from build123d import *

# Parameters (mm, degrees)
F0_W     = 1.5
F0_H     = 2
F0_H_2   = 1.5
F0_W_2   = 6.5
F0_W_3   = 9.5
F1_DEPTH = 89
F2_R     = 1.25
F3_DEPTH = 25


with BuildPart() as f1:
    # F0 (on Front) → F1 (new body)
    with BuildSketch(Plane.XZ):
        with Locations((3.25, -1.75)):
            Rectangle(F0_W, F0_H)
        with Locations((3.25, 0)):
            Rectangle(F0_W, F0_H_2)
        Polygon((4.75, -1.75), (4, -0.75), (4, -2.75), align=None)
        with Locations((-0.75, 0)):
            Rectangle(F0_W_2, F0_H_2)
        with Locations((8.75, -3.5)):
            Rectangle(F0_W_3, F0_H_2)
        with Locations((3.25, -3.5)):
            Rectangle(F0_W, F0_H_2)
        with Locations((14.25, -1.75)):
            Rectangle(F0_W, F0_H)
        with Locations((14.25, -3.5)):
            Rectangle(F0_W, F0_H_2)
        Polygon((12.75, -1.75), (13.5, -2.75), (13.5, -0.75), align=None)
    extrude(amount=-F1_DEPTH)

    # F2 (on face) → F3 (cut)
    with BuildSketch(Plane.XY.offset(0.75)):
        with Locations((0, 4)):
            Circle(F2_R)
        with Locations((0, 85)):
            Circle(F2_R)
    extrude(amount=-F3_DEPTH, mode=Mode.SUBTRACT)


solid = f1.part
Can you work these out from the model? Positions are in its coordinate system, mm. A direction names the side the tool comes from. Round coordinates to 2 decimals unless told otherwise and drop trailing zeros. Write each loop counter-clockwise with the first axis right and the second up, starting at its lowest first coordinate (ties: lowest second). Pieces come first, ordered by that corner, then holes. Notation, with made-up numbers: (62, 7.5) -> (110, 7.5) arc R16 ccw to (110, 18.5) -> close; hole circle Ø7 at (9, -14). An arc over 180 degrees is marked (long way). Use one line per item in the form item = value. Start each with the question number.
Q1. Which directions (+Z, -Z, +X, -X, +Y, -Y) give clear straight access to the entire face, cutting with the end or side of a thin tool? Please do faces 4 (the face through (2.5, 44, -2)), 5 (the face through (5, 0, -3)), 6 (the face through (4, 44, 0)).
Q2. Imagine slicing it at C-C (y = 29.5). Please give me the cut outline in (x, z), then the cut area to 4 significant figures.
Q3. Imagine slicing it at B-B (x = 0). Please give me the cut outline in (y, z), then the cut area to 3 significant figures.
Q4. I'm going to push flat-ended pins straight in: P1, Ø5, axis at x = -1, y = 58.5, coming from the -Z side; P2, Ø1.8, axis at y = 59.5, z = -2.5, coming from the -X side; P3, Ø1.6, axis at x = 14, y = 42, coming from the +Z side. Where does each tip first touch, or does it pass through?
Q5. Imagine slicing it at D-D (x = 7). Please give me the cut outline in (y, z).
Q6. We'd pull the mould along X, two halves only. Please class faces 1 (the face through (-0.27, 2.78, 0.01)), 2 (the face through (15, 44, -3)), 3 (the face through (0, 44, 0.75)): +X half, -X half, draft (parallel to the pull), parting line (faces both ways), or undercut.
Q7. If I drill on probe 1 along Y at (x, z) = (0, -0.2); probe 2 along X at (y, z) = (85, 0); probe 3 along Z at (x, y) = (1.5, 12), over which ranges is the centre line in solid material (lowest first)? Write a range as [from, to].
Q8. Imagine slicing it at A-A (y = 85). Please give me the cut outline in (x, z), then the cut area to 3 significant figures.
Worked out:
q1.face_4 = -Z, -X, +Y, -Y
q1.face_5 = +Z, -Z, +X, -X, -Y
q1.face_6 = +Z, +X, +Y, -Y
q2.outline = (-4, -0.75) -> (2.5, -0.75) -> (2.5, -4.25) -> (15, -4.25) -> (15, -0.75) -> (13.5, -0.75) -> (12.75, -1.75) -> (13.5, -2.75) -> (4, -2.75) -> (4.75, -1.75) -> (4, -0.75) -> (4, 0.75) -> (-4, 0.75) -> close
q2.area = 38.25 mm^2
q3.outline = (0, -0.75) -> (2.75, -0.75) -> (2.75, 0.75) -> (0, 0.75) -> close; (5.25, -0.75) -> (83.75, -0.75) -> (83.75, 0.75) -> (5.25, 0.75) -> close; (86.25, -0.75) -> (89, -0.75) -> (89, 0.75) -> (86.25, 0.75) -> close
q3.area = 126 mm^2
q4.P1 = -0.75
q4.P2 = 2.5
q4.P3 = -0.75
q5.outline = (0, -4.25) -> (89, -4.25) -> (89, -2.75) -> (0, -2.75) -> close
q6.face_1 = undercut
q6.face_2 = +X half
q6.face_3 = draft
q7.probe_1 = [0, 2.75], [5.25, 83.75], [86.25, 89]
q7.probe_2 = [-4, -1.25], [1.25, 4]
q7.probe_3 = [-0.75, 0.75]
q8.outline = (-4, -0.75) -> (-1.25, -0.75) -> (-1.25, 0.75) -> (-4, 0.75) -> close; (1.25, -0.75) -> (2.5, -0.75) -> (2.5, -4.25) -> (15, -4.25) -> (15, -0.75) -> (13.5, -0.75) -> (12.75, -1.75) -> (13.5, -2.75) -> (4, -2.75) -> (4.75, -1.75) -> (4, -0.75) -> (4, 0.75) -> (1.25, 0.75) -> close
q8.area = 34.5 mm^2
